Model file for the job. Use its own axes, mm. A direction names the side the tool comes from. Coordinates: 2 decimals unless noted, no trailing zeros. Write each loop counter-clockwise with the first axis right and the second up, starting at its lowest first coordinate (ties: lowest second). Pieces come first, ordered by that corner, then holes. Notation, with made-up numbers: M 18.25,-31 L 24.25,-31 A28 ccw 24.25,8 Z; hole C -10,72.25 d5. An arc over 180 degrees is marked long. Put each result on its own line as item: value. Start each with the question number.
Q1. Cut at D-D (y = 57). Write the cut outline in (x, z), then the cut area to 3 significant figures.
Q2. Drop flat-ended pins along their axis: pin 1 (3 mm diameter, centred on x = -16, y = 32, fed in from -Z); pin 2 (4 mm diameter, centred on x = -16.5, y = 9.5, fed in from -Z); pin 3 (5 mm diameter, centred on x = 2, z = 26.5, fed in from -Y). Give the stop position or say it passes through.
Q3. Cut at A-A (z = 14). Write the cut outline in (x, y).
Q4. Which spindle directions (+Z, -Z, +X, -X, +Y, -Y) get a long thin tool onto all of the face, cutting with end or side? Do faces 4 (the flat face through (15, 52.8, 0)), 5 (the cylindrical face through (-0.33, 2.12, 7.493)), 6 (the cylindrical face through (7, 12.3, 24.9)), 7 (the flat face through (0, -0.3, 0)), 8 (the flat face through (0, 12, 30)). Say none if no direction does.
Q5. Cut at B-B (y = 9). Write the cut outline in (x, z).
Q6. Pull direction X, two halves, no side cores. Call faces 1 (the cylindrical face through (16.483, 55.335, -0.26)), 2 (the flat face through (-2, 62.2, 2)), 3 (the cylindrical face through (-0.33, 59.969, 7.493)): pulls with the +X half, pulls with the -X half, needs draft (parallel to the pull), parting line crosses it, or undercut.
Q7. Cut at C-C (x = -14.5). Write the cut outline in (y, z).
Q8. Drill centre lines: line 1 along X through (y, z) = (56, 0); line 2 along Y through (x, z) = (4.5, 9.5); line 3 along Z through (x, y) = (-14, 54). Where is each one in solid material? Low to high.
```python
from build123d import *

# Parameters (mm, degrees)
SKETCH_1_R          = 7.5
EXTRUDE_1_DEPTH     = 4.3
SKETCH_2_R          = 21.05
EXTRUDE_2_DEPTH     = 53.5
SKETCH_3_R          = 7.5
EXTRUDE_3_DEPTH     = 4.4
SKETCH_5_R          = 22.5
EXTRUDE_5_DEPTH     = 27
SKETCH_6_R          = 2.5
EXTRUDE_6_DEPTH     = 70
SKETCH_7_R          = 2
CUT_EXTRUDE_1_DEPTH = 5
CHAMFER_1_SIZE      = 0.1
EXTRUDE_7_DEPTH     = 30


with BuildPart() as part:
    # ｽｹｯﾁ1 → ﾎﾞｽ - 押し出し1 (new body)
    with BuildSketch(Plane(origin=(0, 0, 0), x_dir=(1, 0, 0), z_dir=(0, 1, 0))):
        with Locations(Location((0, 0, 0), (0, 0, 90))):
            Circle(SKETCH_1_R)
    extrude(amount=EXTRUDE_1_DEPTH)

    # ｽｹｯﾁ2 → ﾎﾞｽ - 押し出し2 (add)
    with BuildSketch(Plane(origin=(0, 4.3, 0), x_dir=(1, 0, 0), z_dir=(0, 1, 0))):
        with Locations(Location((0, 0, 0), (0, 0, 270))):
            Circle(SKETCH_2_R)
    extrude(amount=EXTRUDE_2_DEPTH)

    # ｽｹｯﾁ3 → ﾎﾞｽ - 押し出し3 (add)
    with BuildSketch(Plane(origin=(0, 57.8, 0), x_dir=(1, 0, 0), z_dir=(0, 1, 0))):
        with Locations(Location((0, 0, 0), (0, 0, 90))):
            Circle(SKETCH_3_R)
    extrude(amount=EXTRUDE_3_DEPTH)

    # ｽｹｯﾁ5 → ﾎﾞｽ - 押し出し5 (add)
    with BuildSketch(Plane(origin=(0, 52.9, 0), x_dir=(1, 0, 0), z_dir=(0, 1, 0))):
        with Locations(Location((0, 0, 0), (0, 0, 270))):
            Circle(SKETCH_5_R)
    extrude(amount=-EXTRUDE_5_DEPTH)

    # ｽｹｯﾁ6 → ﾎﾞｽ - 押し出し6 (add)
    with BuildSketch(Plane(origin=(0, 69.7, 0), x_dir=(1, 0, 0), z_dir=(0, 1, 0))):
        with Locations(Location((0, 0, 0), (0, 0, 270))):
            Circle(SKETCH_6_R)
    extrude(amount=-EXTRUDE_6_DEPTH)

    # ｽｹｯﾁ7 → ｶｯﾄ - 押し出し1 (cut)
    with BuildSketch(Plane(origin=(0, 57.8, 0), x_dir=(1, 0, 0), z_dir=(0, 1, 0))):
        with Locations(Location((14.5, 0, 0), (0, 0, 270))):
            Circle(SKETCH_7_R)
        with Locations(Location((-14.5, 0, 0), (0, 0, 270))):
            Circle(SKETCH_7_R)
    extrude(amount=-CUT_EXTRUDE_1_DEPTH, mode=Mode.SUBTRACT)

    # 面取り1
    chamfer_1_edges = [part.edges().sort_by_distance(p)[0] for p in [
        (0, -0.3, -2.5),
        (0, 69.7, -2.5),
    ]]
    chamfer(chamfer_1_edges, length=CHAMFER_1_SIZE)

    # ｽｹｯﾁ8 → ﾎﾞｽ - 押し出し7 (add)
    with BuildSketch(Plane.XY):
        with BuildLine():
            Line((-5, 14.3), (5, 14.3))
            ThreePointArc((5, 14.3), (7, 12.3), (5, 10.3))
            Line((5, 10.3), (-5, 10.3))
            ThreePointArc((-5, 10.3), (-7, 12.3), (-5, 14.3))
        make_face()
    extrude(amount=EXTRUDE_7_DEPTH)


solid = part.part
```
Computed values:
1. outline: C 0,0 d42.1; hole C -14.5,0 d4; hole C 14.5,0 d4
1. area: 1,370 mm2
2. pin 1: z = -17.2
2. pin 2: z = -15.26
2. pin 3: y = 10.3
3. outline: M -17.61,25.9 L -15.72,25.9 L -15.72,4.3 L 15.72,4.3 L 15.72,25.9 L 17.61,25.9 L 17.61,52.9 L 15.72,52.9 L 15.72,57.8 L -15.72,57.8 L -15.72,52.9 L -17.61,52.9 Z
4. face 4: +Y
4. face 5: -Y
4. face 6: +Z, +X
4. face 7: +Z, -Z, +X, -X, -Y
4. face 8: +Z, +X, -X, +Y, -Y
5. outline: C 0,0 d42.1
6. face 1: undercut
6. face 2: needs draft
6. face 3: parting line crosses it
7. outline: M 4.3,-15.26 L 25.9,-15.26 L 25.9,-17.2 L 52.9,-17.2 L 52.9,-15.26 L 57.8,-15.26 L 57.8,-2 L 52.8,-2 L 52.8,2 L 57.8,2 L 57.8,15.26 L 52.9,15.26 L 52.9,17.2 L 25.9,17.2 L 25.9,15.26 L 4.3,15.26 Z
8. line 1: -21.05 to -16.5, -12.5 to 12.5, 16.5 to 21.05
8. line 2: 4.3 to 57.8
8. line 3: -15.72 to -1.94, 1.94 to 15.72
